Here's how the part is built. I have some questions about the finished solid (model axes, mm). Face numbers are marked on the shaded views. A direction names the side the tool comes from. Round coordinates to 2 decimals unless told otherwise and drop trailing zeros. Loops run counter-clockwise (first coordinate to the right, second up) from the corner with the lowest first, then second, coordinate; pieces in that order, holes last. Notation, with made-up numbers: M 39.25,87.5 L 77.25,87.5 A31 ccw 77.25,111.5 Z; hole C -19.75,-30 d8. An arc over 180 degrees is marked long. Use a Markdown table: item, result.
from build123d import *

# Parameters (mm, degrees)
HIERRO_ANGULAR_2_X_2_X_0_125_1_DEPTH = 126.72
CROQUIS3_W                           = 126.72
CROQUIS3_H                           = 38.8
CORTAR_EXTRUIR1_DEPTH                = 3.175


with BuildPart() as part:
    # Sketch1 → Hierro angular 2 X 2 X 0.125(1) (new body)
    with BuildSketch(Plane(origin=(-63.36, 0, 0), x_dir=(0, -1, 0), z_dir=(1, 0, 0))):
        with BuildLine():
            Line((0, 0), (0, 50.8))
            Line((0, 50.8), (0.00508, 50.8))
            ThreePointArc((0.00508, 50.8), (2.246551928, 49.871551928), (3.175, 47.63008))
            Line((3.175, 47.63008), (3.175, 7.9375))
            ThreePointArc((3.175, 7.9375), (4.569903955, 4.569903955), (7.9375, 3.175))
            Line((7.9375, 3.175), (47.63008, 3.175))
            ThreePointArc((47.63008, 3.175), (49.871551928, 2.246551928), (50.8, 0.00508))
            Line((50.8, 0.00508), (50.8, 0))
            Line((50.8, 0), (0, 0))
        make_face()
    extrude(amount=HIERRO_ANGULAR_2_X_2_X_0_125_1_DEPTH)

    # Croquis3 → Cortar-Extruir1 (cut)
    with BuildSketch(Plane(origin=(0, 0, 0), x_dir=(1, 0, 0), z_dir=(0, 1, 0))):
        with Locations((0, 31.4)):
            Rectangle(CROQUIS3_W, CROQUIS3_H)
    extrude(amount=-CORTAR_EXTRUIR1_DEPTH, mode=Mode.SUBTRACT)


solid = part.part
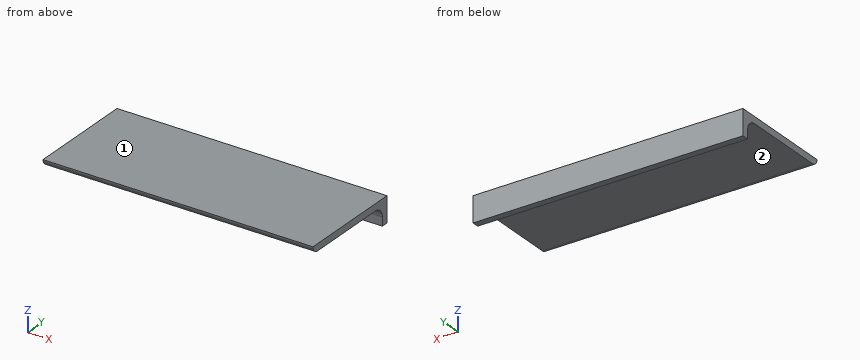
1. Which directions (+Z, -Z, +X, -X, +Y, -Y) give clear straight access to the entire face, cutting with the end or side of a thin tool? Please do the marked faces 1 and 2.
Answer sheet:
| item | result |
|---|---|
| face 1 | +Z, +X, -X, +Y, -Y |
| face 2 | -Z, +X, -X, -Y |
2. I need wall thicknesses on probe 1 along Y at (x, z) = (19.5, -11) (3 decimals); probe 2 along Z at (x, y) = (15.5, -48); probe 3 along Y at (x, z) = (-45.5, -4.75). Which ranges of each line are inside material? Lowest first, please. Write a range as from..to.
Answer sheet:
| item | result |
|---|---|
| probe 1 | -3.175..0 |
| probe 2 | -3.15..0 |
| probe 3 | -4.4..0 |
3. For pin 1 Ø4.5 at (x, z) = (-22, -9.5) entering from -Y, with a flat end and sliding along its axis, tell me the tip position at first contact or that it passes through.
Answer sheet:
| item | result |
|---|---|
| pin 1 | y = -3.22 |
4. Imagine slicing it at B-B, the plane y = -14.5. Write out the boundary of the cut face in (x, z) (3 decimals), then the cut area to 3 significant figures.
Answer sheet:
| item | result |
|---|---|
| outline | M -63.36,-3.175 L 63.36,-3.175 L 63.36,0 L -63.36,0 Z |
| area | 402 mm2 |
